Verification items for the finished model (mm, model axes). A direction names the side the tool comes from. Round coordinates to 2 decimals unless told otherwise and drop trailing zeros. Write each loop counter-clockwise with the first axis right and the second up, starting at its lowest first coordinate (ties: lowest second). Pieces come first, ordered by that corner, then holes. Notation, with made-up numbers: (9.5, 58) - (56.5, 58) arc R24 cw to (56.5, 70) - close; hole circle Ø2 at (82.25, -10.75). An arc over 180 degrees is marked (long way). Answer as a JSON object with one key per item and string values.
Autodesk Inventor part; units mm, degrees
ref_plane "YZ Plane" through (0, 0, 0) normal (1, 0, 0) x (0, 1, 0)
ref_plane "XZ Plane" through (0, 0, 0) normal (0, 1, 0) x (-1, 0, 0)
ref_plane "XY Plane" through (0, 0, 0) normal (0, 0, 1) x (1, 0, 0)
sketch "Esquisse1" plane through (0, 0, 0) normal (0, 1, 0) x (-1, 0, 0)
  line L0 (7.5, 5) -> (-7.5, 5)
  line L1 (-7.5, 5) -> (-7.5, -5)
  line L2 (-7.5, -5) -> (7.5, -5)
  line L3 (7.5, -5) -> (7.5, 5)
  line L4 (7.5, 5) -> (-7.5, -5) construction
  line L5 (7.5, -5) -> (-7.5, 5) construction
  point P0 (0, 0)
  point P1 (0, 0)
  dimension "d0" = 10
  dimension "d1" = 15
extrude "Extrusion1" add sketch "Esquisse1" along normal blind 2
sketch "Esquisse2" plane through (0, 2, 0) normal (0, 1, 0) x (1, 0, 0)
  line L0 (-7.5, 5) -> (-7.5, -5)
  line L1 (7.5, 5) -> (-7.5, 5)
  line L2 (-7.5, -5) -> (-5.5, -5)
  line L3 (-5.5, -5) -> (-5.5, 5)
  line L4 (-5.5, 5) -> (-7.5, 5)
  line L5 (-7.5, 5) -> (-7.5, -5)
  line L6 (-7.5, -5) -> (7.5, -5)
  line L7 (-3.5, -5) -> (-1.5, -5)
  line L8 (-1.5, -5) -> (-1.5, 5)
  line L9 (-1.5, 5) -> (-3.5, 5)
  line L10 (-3.5, 5) -> (-3.5, -5)
  point P0 (0, 0)
  point P1 (-3.5, 5)
  dimension "d4" = 2
  dimension "d5" = 2
  dimension "d6" = 2
extrude "Extrusion2" add sketch "Esquisse2" along normal blind 10 contours L1 L3 L2 L0 | L1 L8 L6 L10
sketch "Esquisse3" plane through (0, 2, 0) normal (0, 1, 0) x (1, 0, 0)
  circle A0 centre (3.75, 0) radius 1.5
  line L0 (-1.5, -5) -> (7.5, -5)
  line L1 (7.5, 5) -> (-1.5, 5)
  line L2 (0, -5) -> (7.5, 5) construction
  line L3 (7.5, -5) -> (7.5, 5)
  line L4 (0, 5) -> (7.5, -5) construction
  point P0 (0, 0)
  point P1 (3.75, 0)
  dimension "d9" = 3
extrude "Extrusion3" cut sketch "Esquisse3" against normal blind 10
properties part number "TOF_holder_Impression 3D"
Q1. Set-up check for faces 5 (the flat face through (-4, 2, 0)), 6 (the flat face through (0, 0, 0)), 7 (the flat face through (-1.5, 7, 0)): record each of +Z, -Z, +X, -X, +Y, -Y from which the full face is reachable in a straight line by a thin tool's end or side.
Geometry check:
{"face 5": "+Z, -Z, +Y", "face 6": "+Z, -Z, +X, -X, -Y", "face 7": "+Z, -Z, +X, +Y"}
Q2. Section check D-D, the plane z = -3.5. Record the cut outline in (x, y).
Geometry check:
{"outline": "(-7.5, 0) - (7.5, 0) - (7.5, 2) - (-1.5, 2) - (-1.5, 12) - (-3.5, 12) - (-3.5, 2) - (-5.5, 2) - (-5.5, 12) - (-7.5, 12) - close"}
Q3. Material ranges on line 1 along X through (y, z) = (4.25, -1.5); line 2 along Z through (x, y) = (3.75, 0.75); line 3 along X through (y, z) = (1.3, 0), recorded low to high. Write a range as [from, to].
Geometry check:
{"line 1": "x = [-7.5, -5.5], [-3.5, -1.5]", "line 2": "z = [-5, -1.5], [1.5, 5]", "line 3": "x = [-7.5, 2.25], [5.25, 7.5]"}
Q4. Section check B-B, the plane x = 3.75. Record the cut outline in (y, z).
Geometry check:
{"outline": "(0, -5) - (2, -5) - (2, -1.5) - (0, -1.5) - close; (0, 1.5) - (2, 1.5) - (2, 5) - (0, 5) - close"}
Q5. Section check C-C, the plane y = 10. Record the cut outline in (x, z).
Geometry check:
{"outline": "(-7.5, -5) - (-5.5, -5) - (-5.5, 5) - (-7.5, 5) - close; (-3.5, -5) - (-1.5, -5) - (-1.5, 5) - (-3.5, 5) - close"}
Q6. Gauge pin test, flat ends, axial feed: P1, Ø1.5, axis at y = 8.5, z = -2, coming from the +X side; P2, Ø2, axis at x = 1, z = 1, coming from the +Y side; P3, Ø6, axis at x = 1, y = 4, coming from the +Z side. Record the tip position at first contact, or that the pin passes through.
Geometry check:
{"P1": "stops at x = -1.5", "P2": "stops at y = 2", "P3": "stops at z = 5"}
Q7. Section check A-A, the plane z = 0. Record the cut outline in (x, y).
Geometry check:
{"outline": "(-7.5, 0) - (2.25, 0) - (2.25, 2) - (-1.5, 2) - (-1.5, 12) - (-3.5, 12) - (-3.5, 2) - (-5.5, 2) - (-5.5, 12) - (-7.5, 12) - close; (5.25, 0) - (7.5, 0) - (7.5, 2) - (5.25, 2) - close"}
Q8. Release check for a two-part mould opening along Z. For faces 1 (the flat face through (-2, 5, 5)), 2 (the flat face through (-2, 5, -5)), 3 (the flat face through (2, 2, 0)), 4 (the cylindrical face through (5.136, 1.014, 0.575)) record: released by +Z, released by -Z, zero draft, split by the parting line, or undercut.
Geometry check:
{"face 1": "released by +Z", "face 2": "released by -Z", "face 3": "zero draft", "face 4": "undercut"}
